Design review of the part built by this model. Coordinates are the model's own, in mm. Coordinates: 2 decimals unless noted, no trailing zeros. Write each loop counter-clockwise with the first axis right and the second up, starting at its lowest first coordinate (ties: lowest second). Pieces come first, ordered by that corner, then holes. Notation, with made-up numbers: M 70,6 L 90,6 A14 ccw 90,16 Z; hole C 61.5,-15.75 d10. An arc over 180 degrees is marked long. Write item = value, one per line.
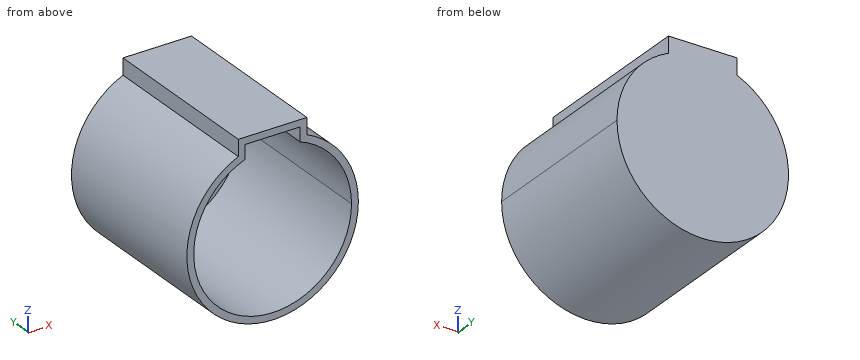
```python
from build123d import *

# Parameters (mm, degrees)
F1_DEPTH = 63.5
F2_T     = -2.54


with BuildPart() as f1:
    # F0 (on Front) → F1 (new body)
    with BuildSketch(Plane.XZ):
        with BuildLine():
            ThreePointArc((-12.7, 29.099355663), (0, 31.75), (12.7, 29.099355663))
            Line((12.7, 29.099355663), (12.7, 35.1254418492))
            Line((12.7, 35.1254418492), (-12.7, 35.1254418492))
            Line((-12.7, 35.1254418492), (-12.7, 29.099355663))
        make_face()
        with BuildLine():
            ThreePointArc((-12.7, 29.099355663), (-17.3901912008, -26.5639558425), (31.75, 0))
            ThreePointArc((31.75, 0), (26.5639558425, 17.3901912008), (12.7, 29.099355663))
            Line((12.7, 29.099355663), (12.7, 28.3745581508))
            Line((12.7, 28.3745581508), (6.3699584668, 28.3745581508))
            ThreePointArc((6.3699584668, 28.3745581508), (22.7039126469, 18.1720739499), (29.0807826772, 0))
            ThreePointArc((29.0807826772, 0), (-18.1720739499, -22.7039126469), (-6.3699584668, 28.3745581508))
            Line((-6.3699584668, 28.3745581508), (-12.7, 28.3745581508))
            Line((-12.7, 28.3745581508), (-12.7, 29.099355663))
        make_face()
        with BuildLine():
            ThreePointArc((29.0807826772, 0), (22.7039126469, 18.1720739499), (6.3699584668, 28.3745581508))
            Line((6.3699584668, 28.3745581508), (-6.3699584668, 28.3745581508))
            ThreePointArc((-6.3699584668, 28.3745581508), (-18.1720739499, -22.7039126469), (29.0807826772, 0))
        make_face()
        with BuildLine():
            Line((-6.3699584668, 28.3745581508), (6.3699584668, 28.3745581508))
            ThreePointArc((6.3699584668, 28.3745581508), (0, 29.0807826772), (-6.3699584668, 28.3745581508))
        make_face()
        with BuildLine():
            Line((12.7, 28.3745581508), (12.7, 29.099355663))
            ThreePointArc((12.7, 29.099355663), (0, 31.75), (-12.7, 29.099355663))
            Line((-12.7, 29.099355663), (-12.7, 28.3745581508))
            Line((-12.7, 28.3745581508), (-6.3699584668, 28.3745581508))
            ThreePointArc((-6.3699584668, 28.3745581508), (0, 29.0807826772), (6.3699584668, 28.3745581508))
            Line((6.3699584668, 28.3745581508), (12.7, 28.3745581508))
        make_face()
    extrude(amount=F1_DEPTH)

    # F2
    f2_openings = [f1.faces().sort_by_distance(p)[0] for p in [
        (0, -63.5, 1.083948),
    ]]
    offset(amount=F2_T, openings=f2_openings, kind=Kind.INTERSECTION)


solid = f1.part
```
Q1. Consider section A-A, the plane y = -41. State the section outline as (x, z) points.
Check result:
outline = M -12.7,29.1 A31.75 ccw long 12.7,29.1 L 12.7,35.13 L -12.7,35.13 Z; hole M -10.16,27.39 A29.21 ccw long 10.16,27.39 L 10.16,32.59 L -10.16,32.59 Z
Q2. Consider section C-C, the plane z = -16. State the section outline as (x, y) points, and give its area (3 significant figures).
Check result:
outline = M -27.42,-63.5 L -24.44,-63.5 L -24.44,-2.54 L 24.44,-2.54 L 24.44,-63.5 L 27.42,-63.5 L 27.42,0 L -27.42,0 Z
area = 503 mm²
Q3. Consider section B-B, the plane x = 0. State the section outline as (y, z) points.
Check result:
outline = M -63.5,-31.75 L 0,-31.75 L 0,35.13 L -63.5,35.13 L -63.5,32.59 L -2.54,32.59 L -2.54,-29.21 L -63.5,-29.21 Z
Q4. For P1, Ø5, axis at y = -33, z = 32, coming from the +X side; P2, Ø5, axis at x = -4, y = -31, coming from the -Z side; P3, Ø3, axis at y = -23.5, z = 31, coming from the -X side, all flat-tipped, find the tip position at first contact; note any pin that passes through.
Check result:
P1 = 12.7
P2 = -31.71
P3 = -12.7
Q5. Wall thickness on line 1 (Z direction, x = 0, y = -25.5); line 2 (Y direction, x = -27, z = 4.5); line 3 (X direction, y = -38, z = 6): over which ranges is each line inside the solid? List them lowest first.
Check result:
line_1 = -31.75 to -29.21, 32.59 to 35.13
line_2 = -2.54 to 0
line_3 = -31.18 to -28.59, 28.59 to 31.18
